Can you work these out from the model? Positions are in its coordinate system, mm. A direction names the side the tool comes from. Round coordinates to 2 decimals unless told otherwise and drop trailing zeros. Write each loop counter-clockwise with the first axis right and the second up, starting at its lowest first coordinate (ties: lowest second). Pieces come first, ordered by that corner, then holes. Notation, with made-up numbers: (67.5, -22) - (71.5, -22) arc R25 ccw to (71.5, 16) - close; hole circle Ø1 at (30, -13). An arc over 180 degrees is marked (long way). One line per item, written item: value. Start each with the question number.
(1) I want a section at B-B on x = -26. List the corners of the cut face in (y, z) for me, plus the area to 3 significant figures.
(2) If I drill on L1, parallel to Z at x = -61, y = 0.2; L2, parallel to Z at x = -40, y = 1.4; L3, parallel to X at y = 0.1, z = -22, over which ranges is the centre line in solid material (lowest first)? Write a range as from..to.
(3) Thinking about a two-plate mould opening in Z: for faces 1 (the face through (-22, 0, 0)), 2 (the face through (-18, 1, 33)), 3 (the face through (18, 1, 6)), which applies, +Z half, -Z half, draft (parallel to the pull), parting line (faces both ways), or undercut?
(4) On a 3-axis mill with a long thin cutter (end or side, diameter ignored), from which of +Z, -Z, +X, -X, +Y, -Y can I reach the whole of each face in a straight line? I mean faces 4 (the face through (-22, 2.5, 0)), 5 (the face through (-29, 1, 26)). Say none if no direction works.
(5) I want a section at A-A on z = 15.5. List the corners of the cut face in (x, y) for me, plus the area to 3 significant figures.
(6) I want a section at C-C on y = 0.95. Give the number of separate pieces and of enclosed holes in the cut face, plus the area to 3 significant figures.
from build123d import *

# Parameters (mm, degrees)
SKETCH1_W           = 160
SKETCH1_H           = 66
BOSS_EXTRUDE1_DEPTH = 40
SKETCH2_R           = 4.025
SKETCH2_W           = 130
SKETCH2_H           = 37.5
CUT_EXTRUDE1_DEPTH  = 112.157545853
SKETCH3_R           = 1
SKETCH3_W           = 120
SKETCH3_H           = 20
CUT_EXTRUDE2_DEPTH  = 96.336247042
SKETCH4_R           = 12.5
CUT_EXTRUDE3_DEPTH  = 95.314633011
SKETCH5_W           = 35
SKETCH5_H           = 66
CUT_EXTRUDE5_DEPTH  = 96.336247042


with BuildPart() as part:
    # Sketch1 → Boss-Extrude1 (new body)
    with BuildSketch(Plane(origin=(0, 0, 0), x_dir=(1, 0, 0), z_dir=(0, 1, 0))):
        Rectangle(SKETCH1_W, SKETCH1_H)
    extrude(amount=BOSS_EXTRUDE1_DEPTH)

    # Sketch2 → Cut-Extrude1 (cut, through all)
    with BuildSketch(Plane.XY.offset(33)):
        with Locations((70, 20)):
            Circle(SKETCH2_R)
        with Locations((-15, 21.25)):
            Rectangle(SKETCH2_W, SKETCH2_H)
    extrude(amount=-CUT_EXTRUDE1_DEPTH, mode=Mode.SUBTRACT)

    # Sketch3 → Cut-Extrude2 (cut, through all)
    with BuildSketch(Plane(origin=(0, 40, 0), x_dir=(1, 0, 0), z_dir=(0, 1, 0))):
        with Locations(Location((-75, 29.5, 0), (0, 0, 270))):
            Circle(SKETCH3_R)
        with Locations(Location((-75, 2.5, 0), (0, 0, 270))):
            Circle(SKETCH3_R)
        with Locations(Location((-67, 29.5, 0), (0, 0, 270))):
            Circle(SKETCH3_R)
        with Locations(Location((-59, 29.5, 0), (0, 0, 270))):
            Circle(SKETCH3_R)
        with Locations(Location((-51, 29.5, 0), (0, 0, 270))):
            Circle(SKETCH3_R)
        with Locations(Location((-67, 2.5, 0), (0, 0, 270))):
            Circle(SKETCH3_R)
        with Locations(Location((-59, 2.5, 0), (0, 0, 270))):
            Circle(SKETCH3_R)
        with Locations(Location((-51, 2.5, 0), (0, 0, 270))):
            Circle(SKETCH3_R)
        with Locations(Location((-6.5, 29.5, 0), (0, 0, 270))):
            Circle(SKETCH3_R)
        with Locations(Location((-6.5, 2.5, 0), (0, 0, 270))):
            Circle(SKETCH3_R)
        with Locations(Location((1.5, 29.5, 0), (0, 0, 270))):
            Circle(SKETCH3_R)
        with Locations(Location((9.5, 29.5, 0), (0, 0, 270))):
            Circle(SKETCH3_R)
        with Locations(Location((17.5, 29.5, 0), (0, 0, 270))):
            Circle(SKETCH3_R)
        with Locations(Location((1.5, 2.5, 0), (0, 0, 270))):
            Circle(SKETCH3_R)
        with Locations(Location((9.5, 2.5, 0), (0, 0, 270))):
            Circle(SKETCH3_R)
        with Locations(Location((17.5, 2.5, 0), (0, 0, 270))):
            Circle(SKETCH3_R)
        with Locations((17.5, -2.5)):
            Circle(SKETCH3_R)
        with Locations((9.5, -2.5)):
            Circle(SKETCH3_R)
        with Locations((1.5, -2.5)):
            Circle(SKETCH3_R)
        with Locations((17.5, -29.5)):
            Circle(SKETCH3_R)
        with Locations((9.5, -29.5)):
            Circle(SKETCH3_R)
        with Locations((1.5, -29.5)):
            Circle(SKETCH3_R)
        with Locations((-6.5, -2.5)):
            Circle(SKETCH3_R)
        with Locations((-6.5, -29.5)):
            Circle(SKETCH3_R)
        with Locations((-51, -2.5)):
            Circle(SKETCH3_R)
        with Locations((-59, -2.5)):
            Circle(SKETCH3_R)
        with Locations((-67, -2.5)):
            Circle(SKETCH3_R)
        with Locations((-51, -29.5)):
            Circle(SKETCH3_R)
        with Locations((-59, -29.5)):
            Circle(SKETCH3_R)
        with Locations((-67, -29.5)):
            Circle(SKETCH3_R)
        with Locations((-75, -2.5)):
            Circle(SKETCH3_R)
        with Locations((-75, -29.5)):
            Circle(SKETCH3_R)
        with Locations((-17.5, 16)):
            Rectangle(SKETCH3_W, SKETCH3_H)
        with Locations((-17.5, -16)):
            Rectangle(SKETCH3_W, SKETCH3_H)
    extrude(amount=-CUT_EXTRUDE2_DEPTH, mode=Mode.SUBTRACT)

    # Sketch4 → Cut-Extrude3 (cut, through all)
    with BuildSketch(Plane(origin=(0, 2.5, 0), x_dir=(1, 0, 0), z_dir=(0, 1, 0))):
        with Locations((-44.25, -16)):
            Circle(SKETCH4_R)
        with Locations((-44.25, 16)):
            Circle(SKETCH4_R)
        with Locations((-13.25, 16)):
            Circle(SKETCH4_R)
        with Locations((-13.25, -16)):
            Circle(SKETCH4_R)
    extrude(amount=-CUT_EXTRUDE3_DEPTH, mode=Mode.SUBTRACT)

    # Sketch5 → Cut-Extrude5 (cut, through all)
    with BuildSketch(Plane(origin=(0, 40, 0), x_dir=(1, 0, 0), z_dir=(0, 1, 0))):
        with Locations((62.5, 0)):
            Rectangle(SKETCH5_W, SKETCH5_H)
    extrude(amount=-CUT_EXTRUDE5_DEPTH, mode=Mode.SUBTRACT)


solid = part.part
Established:
1. outline: (0, -33) - (2.5, -33) - (2.5, -26) - (0, -26) - close; (0, -6) - (2.5, -6) - (2.5, 6) - (0, 6) - close; (0, 26) - (2.5, 26) - (2.5, 33) - (0, 33) - close
1. area: 65.0 mm2
2. L1: -33..-26, -6..6, 26..33
2. L2: -33..-27.76, -4.24..4.24, 27.76..33
2. L3: -80..-77.5, 42.5..45
3. face 1: draft
3. face 2: +Z half
3. face 3: undercut
4. face 4: +Z, -Z, +X, -X, +Y
4. face 5: +Y, -Y
5. outline: (-80, 0) - (-77.5, 0) - (-77.5, 2.5) - (-80, 2.5) - close; (42.5, 0) - (45, 0) - (45, 2.5) - (42.5, 2.5) - close
5. area: 12.5 mm2
6. separate pieces: 1
6. enclosed holes: 34
6. area: 3,150 mm2
